Input: part model. Units: mm. Frame: model coordinates. A direction names the side the tool comes from. Give positions to 0.01 mm unless a question says otherwise; leave off trailing zeros.
```python
from build123d import *

# Parameters (mm, degrees)
SKETCH1_R           = 0.6
BOSS_EXTRUDE1_DEPTH = 4
FILLET3_R           = 0.1
FILLET4_R           = 0.5
SKETCH6_W           = 5.5
SKETCH6_H           = 1.5
CUT_EXTRUDE3_DEPTH  = 12.5
CHAMFER5_SIZE       = 2
CHAMFER6_SIZE       = 2
CHAMFER7_SIZE       = 3
CHAMFER8_SIZE       = 1


with BuildPart() as part:
    # Sketch1 → Boss-Extrude1 (new body)
    with BuildSketch(Plane.XY):
        with BuildLine():
            Line((0, 27.832467291), (0, 0))
            Line((0, 0), (37.79685519, 0))
            ThreePointArc((37.79685519, 0), (24.974482689, 22.16759606), (0, 27.832467291))
        make_face()
        with Locations((6, 2)):
            Circle(SKETCH1_R, mode=Mode.SUBTRACT)
        with Locations((6, 8)):
            Circle(SKETCH1_R, mode=Mode.SUBTRACT)
        with BuildLine():
            Line((33.211027176, 3), (12, 3))
            Line((12, 3), (31.393734472, 8.19653549))
            ThreePointArc((31.393734472, 8.19653549), (32.430403559, 5.643038878), (33.211027176, 3))
        make_face(mode=Mode.SUBTRACT)
        with BuildLine():
            Line((28.785067971, 12.67392631), (10.80845767, 7.857108097))
            Line((10.80845767, 7.857108097), (25.599351889, 16.396634856))
            ThreePointArc((25.599351889, 16.396634856), (27.273796122, 14.605098147), (28.785067971, 12.67392631))
        make_face(mode=Mode.SUBTRACT)
        with BuildLine():
            ThreePointArc((6.022317364, 16.759671956), (5.519466967, 17.386683928), (5, 18))
            Line((5, 18), (5, 24.382137159))
            ThreePointArc((5, 24.382137159), (8.938861294, 24.245342416), (12.819495121, 23.556849712))
            Line((12.819495121, 23.556849712), (6.022317364, 16.759671956))
        make_face(mode=Mode.SUBTRACT)
        with BuildLine():
            ThreePointArc((18.021652475, 21.687939255), (19.760252022, 20.785558519), (21.431506729, 19.763831023))
            Line((21.431506729, 19.763831023), (8.811215985, 12.477502764))
            Line((8.811215985, 12.477502764), (18.021652475, 21.687939255))
        make_face(mode=Mode.SUBTRACT)
    extrude(amount=BOSS_EXTRUDE1_DEPTH)

    # Fillet3
    fillet3_edges = [part.edges().sort_by_distance(p)[0] for p in [
        (12, 3, 2),
        (10.80845767, 7.857108097, 2),
        (8.811215985, 12.477502764, 2),
    ]]
    fillet(fillet3_edges, radius=FILLET3_R)

    # Fillet4
    fillet4_edges = [part.edges().sort_by_distance(p)[0] for p in [
        (6.022317364, 16.759671956, 2),
        (12.819495121, 23.556849712, 2),
        (5, 24.382137159, 2),
        (5, 18, 2),
        (33.211027176, 3, 2),
        (31.393734472, 8.19653549, 2),
        (28.785067971, 12.67392631, 2),
        (25.599351889, 16.396634856, 2),
        (21.431506729, 19.763831023, 2),
        (18.021652475, 21.687939255, 2),
    ]]
    fillet(fillet4_edges, radius=FILLET4_R)

    # Sketch6 → Cut-Extrude3 (cut)
    with BuildSketch(Plane.XZ):
        with Locations((6, 2)):
            Rectangle(SKETCH6_W, SKETCH6_H)
    extrude(amount=-CUT_EXTRUDE3_DEPTH, mode=Mode.SUBTRACT)

    # Chamfer5
    chamfer5_edges = [part.edges().sort_by_distance(p)[0] for p in [
        (24.974482689, 22.16759606, 0),
    ]]
    chamfer(chamfer5_edges, length=CHAMFER5_SIZE)

    # Chamfer6
    chamfer6_edges = [part.edges().sort_by_distance(p)[0] for p in [
        (24.974482689, 22.16759606, 4),
    ]]
    chamfer(chamfer6_edges, length=CHAMFER6_SIZE - 0.0001)  # a hair under: the kernel refuses the full size

    # Chamfer7
    chamfer7_edges = [part.edges().sort_by_distance(p)[0] for p in [
        (0, 12.896938457, 0),
    ]]
    chamfer(chamfer7_edges, length=CHAMFER7_SIZE)

    # Chamfer8
    chamfer8_edges = [part.edges().sort_by_distance(p)[0] for p in [
        (0, 12.896989488, 4),
    ]]
    chamfer(chamfer8_edges, length=CHAMFER8_SIZE - 0.0001)  # a hair under: the kernel refuses the full size


solid = part.part
```
Item 1: Set-up query: faces 4 (the flat face through (6, 6, 1.25)), 5 (the flat face through (18.271, 12.165, 1.972)), 6 (the flat face through (0.5, 13.6, 3.5)). Return all of +Z, -Z, +X, -X, +Y, -Y with unobstructed straight access to the full face (end or side cutting, diameter ignored); none if empty.
Item 2: Mould query, pull axis X, two halves, no side actions, for faces 1 (the flat face through (14, 10, 4)), 2 (the flat face through (2, 14, 1)), 3 (the cylindrical face through (19.54, 20.91, 1.97)). Classes: +X half, -X half, draft (parallel to the pull), parting line (faces both ways), or undercut.
Item 3: Section A-A (z = 0.6). Give the number of separate pieces and of enclosed holes in the cut face, and give its area (3 significant figures).
Item 4: Ray query, line 1 (Y direction, x = 18, z = 1.35); line 2 (X direction, y = 21, z = 2.1); line 3 (Y direction, x = 6, z = 0.45). Return the intervals inside material, ascending.
Item 5: Pin query (flat end, axial travel): pin 1 (1.2 mm diameter, centred on y = 21.5, z = 2.5, fed in from +X); pin 2 (1 mm diameter, centred on y = 11, z = 0.5, fed in from +X); pin 3 (1.5 mm diameter, centred on x = 31.5, y = 17, fed in from +Z); pin 4 (0.8 mm diameter, centred on y = 3, z = 2, fed in from -X). Return the tip coordinate at first contact, or that it passes through.
Solved:
1. face 4: -Y
1. face 5: +Z, -Z
1. face 6: +Z, -X, +Y, -Y
2. face 1: draft
2. face 2: -X half
2. face 3: undercut
3. separate pieces: 1
3. enclosed holes: 6
3. area: 565 mm2
4. line 1: y = 0 to 3, 4.61 to 9.78, 12.01 to 17.78, 21.57 to 25.36
4. line 2: x = 0.9 to 5, 10.26 to 17.33, 19.37 to 26.31
4. line 3: y = 0 to 1.4, 2.6 to 7.4, 8.6 to 17.01, 24.4 to 26.85
5. pin 1: stops at x = 26.26
5. pin 2: stops at x = 33.41
5. pin 3: passes through
5. pin 4: stops at x = 0.6
